Source: CAD feature listing. Evaluate the final solid. Frame: model axes, mm. Give positions to 0.01 mm unless a question says otherwise; leave off trailing zeros. Order: outer loops, then holes, each group sorted by start corner. A loop starts at its lowest first (then second) coordinate and runs counter-clockwise, first axis right, second up.
```python
from build123d import *

# Parameters (mm, degrees)
SKETCH_2_W          = 900
SKETCH_2_H          = 680
EXTRUDE_1_DEPTH     = 40
HOLE_WIZARD_M5_1_D  = 4.2
HOLE_WIZARD_M5_2_D  = 4.2
SKETCH_9_R          = 12.5
CUT_EXTRUDE_1_DEPTH = 566.420197729


with BuildPart() as part:
    # 草图2 → 凸台-拉伸1 (new body)
    with BuildSketch(Plane.XY):
        Rectangle(SKETCH_2_W, SKETCH_2_H)
    extrude(amount=EXTRUDE_1_DEPTH)

    # M5 螺纹孔1 (through all)
    with Locations(Plane(origin=(0, -340, 0), x_dir=(-1, 0, 0), z_dir=(0, -1, 0))):
        with Locations((0, -20)):
            Hole(HOLE_WIZARD_M5_1_D / 2)

    # M5 螺纹孔2 (through all)
    with Locations(Plane.ZY.offset(450)):
        with Locations((20, 0)):
            Hole(HOLE_WIZARD_M5_2_D / 2)

    # 草图9 → 切除-拉伸1 (cut, through all)
    with BuildSketch(Plane.XY.offset(40)):
        with Locations((-398, 250)):
            Circle(SKETCH_9_R)
    extrude(amount=-CUT_EXTRUDE_1_DEPTH, mode=Mode.SUBTRACT)


solid = part.part
```
1) Draft query along Y for faces 1 (the cylindrical face through (-391.28, 260.54, 20.28)), 2 (the flat face through (-6, 340, 20)), 3 (the flat face through (-6, 5, 40)). Return one class per face: +Y half, -Y half, draft (parallel to the pull), parting line (faces both ways), or undercut.
Report:
face 1: undercut
face 2: +Y half
face 3: draft
2) Section query B-B, the plane y = 250. Return the cut outline in (x, z), and give its area (3 significant figures).
Report:
outline: (-450, 0) - (-410.5, 0) - (-410.5, 40) - (-450, 40) - close; (-385.5, 0) - (450, 0) - (450, 40) - (-385.5, 40) - close; hole circle Ø4.2 at (0, 20)
area: 35,000 mm2
3) Section query A-A, the plane x = -398. Return the cut outline in (y, z).
Report:
outline: (-340, 0) - (237.5, 0) - (237.5, 40) - (-340, 40) - close; (262.5, 0) - (340, 0) - (340, 40) - (262.5, 40) - close; hole circle Ø4.2 at (0, 20)
4) Material intervals for L1, parallel to Y at x = -108, z = 20; L2, parallel to Z at x = 228, y = 0; L3, parallel to Y at x = -398, z = 15, sorted ascending.
Report:
L1: y = -340 to -2.1, 2.1 to 340
L2: z = 0 to 17.9, 22.1 to 40
L3: y = -340 to 237.5, 262.5 to 340
